Answer from the drawing. Dimensions are ordinates in mm from the lowest x, y and z of the part. Coordinates: 2 decimals unless noted, no trailing zeros. Write each loop counter-clockwise with the first axis right and the second up, starting at its lowest first coordinate (ties: lowest second). Pieces come first, ordered by that corner, then holes.
(1) Section D-D on z = 5 is taken. Write down the section's boundary in (x, y), then the cut area to 3 significant figures.
(2) Find the intervals of material crossed by probe 1 along Y at (x, z) = (22, 17.75); probe 2 along X at (y, z) = (24, 10); probe 3 along X at (y, z) = (15.5, 15.5), in increasing order.
(3) Section A-A on x = 22.5 is taken. Write down the section's boundary in (y, z), then the cut area to 3 significant figures.
(4) Given pin 1 (1.5 mm diameter, centred on x = 27, z = 18.5, fed in from -Y); pin 2 (4 mm diameter, centred on x = 16.5, y = 12.5, fed in from -Z); pin 3 (6 mm diameter, centred on y = 6, z = 16, fed in from -X); pin 4 (6 mm diameter, centred on y = 4.5, z = 17.5, fed in from -X), each flat-ended and moving along its own axis, determine where each tip first touches the part or whether it passes through.
(5) Section C-C on z = 20.5 is taken. Write down the section's boundary in (x, y), then the cut area to 3 significant figures.
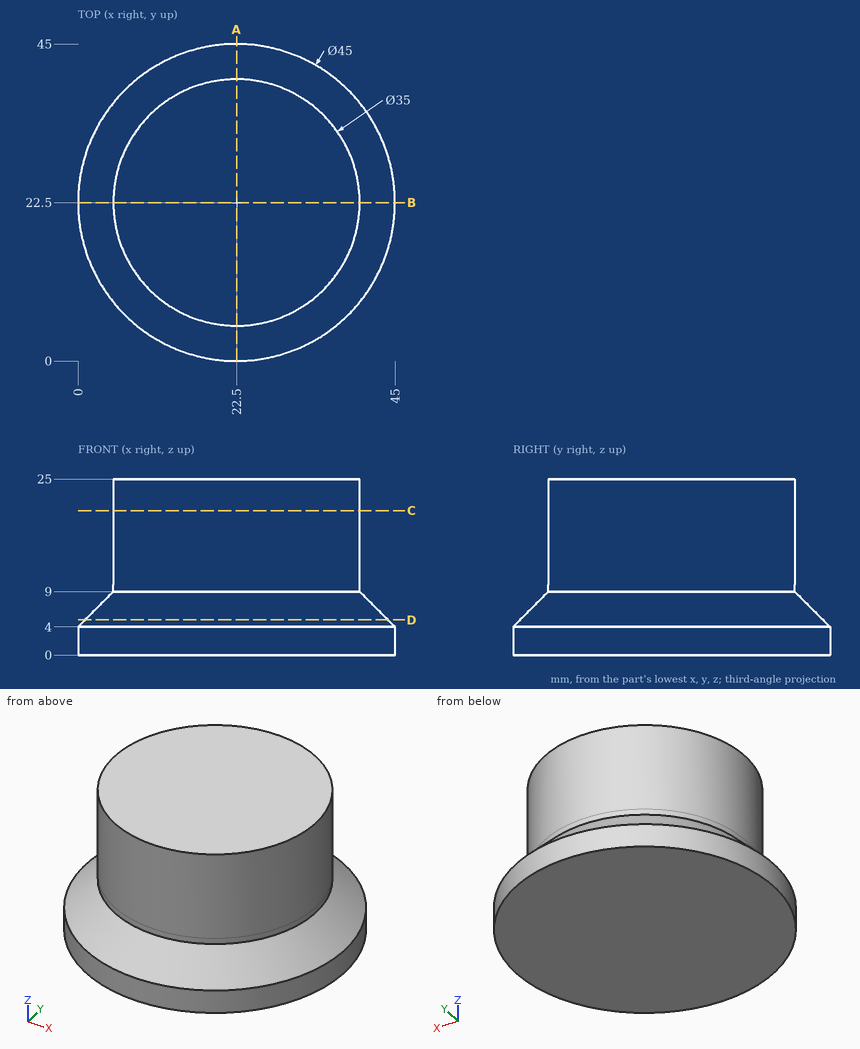
Response:
1. outline: circle Ø43 at (22.5, 22.5)
1. area: 1,450 mm2
2. probe 1: y = 5.01 to 39.99
2. probe 2: x = 5.06 to 39.94
2. probe 3: x = 6.46 to 38.54
3. outline: (0, 0) - (45, 0) - (45, 4) - (40, 9) - (40, 25) - (5, 25) - (5, 9) - (0, 4) - close
3. area: 940 mm2
4. pin 1: stops at y = 5.41
4. pin 2: stops at z = 0
4. pin 3: stops at x = 11.36
4. pin 4: stops at x = 13.49
5. outline: circle Ø35 at (22.5, 22.5)
5. area: 962 mm2
